Autodesk Inventor part; units mm, degrees
ref_plane "YZ Plane" through (0, 0, 0) normal (1, 0, 0) x (0, 1, 0)
ref_plane "XZ Plane" through (0, 0, 0) normal (0, 1, 0) x (-1, 0, 0)
ref_plane "XY Plane" through (0, 0, 0) normal (0, 0, 1) x (1, 0, 0)
sketch "face_sketch" plane through (0, 0, 0) normal (0, 1, 0) x (-1, 0, 0)
  line L0 (0, 0) -> (25.4, 0)
  line L1 (25.4, 0) -> (25.4, -127)
  line L2 (25.4, -127) -> (0, -127)
  line L3 (0, -127) -> (0, 0)
  line L4 (25.4, -50.8) -> (152.4, -50.8)
  line L5 (152.4, -50.8) -> (152.4, -76.2)
  line L6 (152.4, -76.2) -> (25.4, -76.2)
  line L7 (25.4, -76.2) -> (25.4, -50.8)
  line L8 (152.4, -50.8) -> (25.4, 0)
  line L9 (152.4, -76.2) -> (25.4, -127)
  dimension "d0" = 25.4
  dimension "d1" = 127
  dimension "d2" = 127
  dimension "d3" = 25.4
extrude "Plate1" add sketch "face_sketch" along normal blind 3.048
sketch "rivet_holes_sketch" plane through (0, 3.048, 0) normal (0, 1, 0) x (1, 0, 0)
  line L0 (-25.4, 0) -> (-152.4, 50.8)
  line L1 (0, 0) -> (-25.4, 0)
  line L2 (0, 127) -> (0, 0)
  line L3 (-25.4, 127) -> (0, 127)
  line L4 (-152.4, 76.2) -> (-25.4, 127)
  line L5 (-152.4, 50.8) -> (-152.4, 76.2)
  line L6 (-25.4, 127) -> (-25.4, 0) construction
  line L7 (0, 127) -> (-25.4, 127) construction
  line L8 (-25.4, 0) -> (0, 0) construction
  line L9 (-152.4, 76.2) -> (-152.4, 50.8) construction
  line L10 (-152.4, 63.5) -> (-131.2333, 63.5) construction
  line L11 (-131.2333, 63.5) -> (-110.0667, 63.5) construction
  line L12 (-110.0667, 63.5) -> (-88.9, 63.5) construction
  line L13 (-88.9, 63.5) -> (-67.7333, 63.5) construction
  line L14 (-67.7333, 63.5) -> (-46.5667, 63.5) construction
  line L15 (-46.5667, 63.5) -> (-25.4, 63.5) construction
  line L16 (-12.7, 0) -> (-12.7, 21.1667) construction
  line L17 (-12.7, 21.1667) -> (-12.7, 42.3333) construction
  line L18 (-12.7, 42.3333) -> (-12.7, 63.5) construction
  line L19 (-12.7, 63.5) -> (-12.7, 84.6667) construction
  line L20 (-12.7, 84.6667) -> (-12.7, 105.8333) construction
  line L21 (-12.7, 105.8333) -> (-12.7, 127) construction
hole "rivet_holes" at (-131.2333, 3.048, -63.5) at (-110.0667, 3.048, -63.5) at (-88.9, 3.048, -63.5) at (-67.7333, 3.048, -63.5) at (-46.5667, 3.048, -63.5) at (-12.7, 3.048, -21.1667) at (-12.7, 3.048, -42.3333) at (-12.7, 3.048, -63.5) at (-12.7, 3.048, -84.6667) at (-12.7, 3.048, -105.8333) direction (0, -1, 0) diameter 3.5719 depth 3.048 tip angle 118
sketch "hm_mounting_slot_sketch" plane through (0, 3.048, 0) normal (0, 1, 0) x (1, 0, 0)
  line L0 (-67.437, 87.503) -> (-26.797, 87.503) construction
  line L1 (-67.437, 88.9) -> (-26.797, 88.9)
  line L2 (-26.797, 86.106) -> (-67.437, 86.106)
  arc A0 (-67.437, 88.9) -> (-67.437, 86.106) centre (-67.437, 87.503) ccw
  arc A1 (-26.797, 86.106) -> (-26.797, 88.9) centre (-26.797, 87.503) ccw
  line L3 (-67.437, 39.497) -> (-26.797, 39.497) construction
  line L4 (-67.437, 38.1) -> (-26.797, 38.1)
  line L5 (-26.797, 40.894) -> (-67.437, 40.894)
  arc A2 (-67.437, 40.894) -> (-67.437, 38.1) centre (-67.437, 39.497) ccw
  arc A3 (-26.797, 38.1) -> (-26.797, 40.894) centre (-26.797, 39.497) ccw
  line L6 (-25.4, 0) -> (-25.4, 127) construction
  line L7 (-68.834, 87.503) -> (-68.834, 109.6264) construction
  line L8 (-25.4, 127) -> (-152.4, 76.2)
  line L9 (-68.834, 39.497) -> (-68.834, 17.3736) construction
  line L10 (-152.4, 50.8) -> (-25.4, 0)
  point P0 (0, 0)
  point P1 (-47.117, 87.503)
  point P2 (-47.117, 39.497)
  point P3 (-25.4, 39.497)
  point P4 (-25.4, 87.503)
  point P5 (-68.834, 28.4353)
  dimension "d12" = 40.64
  dimension "d14" = 2.794
  dimension "d15" = 40.64
  dimension "d16" = 2.794
  dimension "d17" = 50.8
extrude "Cut1" cut sketch "hm_mounting_slot_sketch" against normal blind 3.048
equation "\"d5\" = rv_hole_diameter"
equation "\"d10\" = Thickness"
equation "\"d12\" = tb_hm_mounting_slot_length"
equation "\"d15\" = tb_hm_mounting_slot_length"
equation "\"d17\" = hm_base_length"
equation "\"d18\" = Thickness"
equation "\"d0\" = st_outer_diameter"
equation "\"d1\" = tb_rivet_row_length"
equation "\"d2\" = tb_rivet_row_length"
equation "\"d3\" = st_outer_diameter"
equation "\"Thickness\" = tb_metal_thickness"
equation "\"BendRadius\" = Thickness"
equation "\"BendReliefWidth\" = Thickness"
equation "\"BendReliefDepth\" = 0.5 * Thickness"
equation "\"CornerReliefSize\" = 4 * Thickness"
equation "\"MinimumRemnant\" = 2 * Thickness"
equation "\"TransitionRadius\" = BendRadius"
equation "\"JacobiRadiusSize\" = BendRadius"
equation "\"GapSize\" = Thickness"
equation "\"bp_thickness\" = 3.048"
equation "\"bp_height\" = gb_mh_seperation + st_outer_diameter"
equation "\"bp_width\" = 4 * st_rivet_distance"
equation "\"bp_axle_height\" = magic_axle_offset + gb_axle_from_edge + gb_to_bottom_of_side_assembly"
equation "\"magic_axle_offset\" = 2.286"
equation "\"bp_tensioner_width\" = 6.35"
equation "\"bp_tensioner_height\" = 50.8"
equation "\"bp_tensioner_from_bottom\" = 38.1"
equation "\"bp_tensioner_from_side\" = 25.4"
equation "\"bp_tensioner_wood_mount_from_tensioner_top\" = 12.7"
equation "\"bp_tensioner_wood_mount_diameter\" = 6.35"
equation "\"gb_mh_seperation\" = 111.1504"
equation "\"gb_mh_diameter\" = 6.35"
equation "\"gb_axle_from_edge\" = 38.1"
equation "\"gb_width\" = 127"
equation "\"gb_bearing_diameter\" = 28.575"
equation "\"gb_to_bottom_of_side_assembly\" = 4.7752"
equation "\"rv_hole_diameter\" = 3.57187"
equation "\"st_outer_diameter\" = 25.4"
equation "\"st_wall_thickness\" = 1.5875"
equation "\"st_length\" = 685.8"
equation "\"st_gbmh_from_center\" = 0.5 * gb_mh_seperation"
equation "\"st_cutout_depth_right\" = 203.2"
equation "\"st_cutout_depth_left\" = 203.2"
equation "\"st_rivet_distance\" = 19.05"
equation "\"so_inner_diameter\" = 7.62"
equation "\"so_wall_thickness\" = 5.08"
equation "\"so_length\" = 40.64"
equation "\"twb_width\" = st_outer_diameter"
equation "\"twb_length\" = bp_tensioner_width + 2 * twb_margin_on_each_side"
equation "\"twb_height\" = 2 * bp_tensioner_wood_mount_diameter + bp_tensioner_height + 2 * bp_tensioner_wood_mount_from_tensioner_top + twb_margin_on_each_side"
equation "\"twb_margin_on_each_side\" = 6.35"
equation "\"twb_tensioner_from_edge\" = -0.5 * bp_tensioner_height + 0.5 * twb_height"
equation "\"tb_side_length\" = 127"
equation "\"tb_rivet_row_length\" = 127"
equation "\"d4\" = BendRadius"
equation "\"tb_metal_thickness\" = 3.048"
equation "\"tb_hm_mounting_slot_length\" = 40.64"
equation "\"hm_base_width\" = 30.48"
equation "\"hm_base_length\" = 50.8"
equation "\"hm_moon_flange_radius\" = 17.78"
equation "\"hm_moon_channel_offset\" = 2.286"
equation "\"hm_moon_flange_width\" = 5.08"
equation "\"hm_moon_thickness\" = 5.08"
equation "\"hm_base_height\" = 5.08"
equation "\"hm_peg_width\" = 2.54"
equation "\"hm_peg_length\" = 5.08"
equation "\"hm_peg_height\" = 5.08"
equation "\"hm_rivet_groove_width\" = 10.16"
equation "\"hm_rivet_groove_height\" = 1.27"
equation "\"gb_mh_seperation_alt\" = 111.125"
equation "\"gb_axle_from_edge_alt\" = 43.1546"
equation "\"bp_axle_height_alt\" = magic_axle_offset + gb_axle_from_edge_alt + gb_to_bottom_of_side_assembly"
properties part number "traingle_bracket(tb)" material "Aluminum 6061"
Source: CAD feature listing. Evaluate the final solid. Frame: model axes, mm. A direction names the side the tool comes from. Round coordinates to 2 decimals unless told otherwise and drop trailing zeros. Order: outer loops, then holes, each group sorted by start corner. A loop starts at its lowest first (then second) coordinate and runs counter-clockwise, first axis right, second up. Notation, with made-up numbers: (-26, 46.25) -> (17, 46.25) arc R33 cw to (17, 75.25) -> close; hole circle Ø4 at (-38, -2). An arc over 180 degrees is marked (long way). Answer as CSV lines item,"result".
Item 1: Pull-direction query (X, two-part tool) for faces 3 (the face through (-89.789, 1.503, -101.244)), 4 (the face through (-13.236, 1.503, -82.963)), 5 (the face through (-14.206, 1.503, -104.873)), 6 (the face through (-58, 0, -63)); classes: pulls with the +X half, pulls with the -X half, needs draft (parallel to the pull), parting line crosses it, or undercut.
A:
face 3,"pulls with the -X half"
face 4,"undercut"
face 5,"undercut"
face 6,"needs draft"
Item 2: Section D-D, the plane x = -41.5. Return loops of the section in (y, z), plus the area to 3 significant figures.
A:
outline,"(0, -120.56) -> (3.05, -120.56) -> (3.05, -88.9) -> (0, -88.9) -> close; (0, -86.11) -> (3.05, -86.11) -> (3.05, -40.89) -> (0, -40.89) -> close; (0, -38.1) -> (3.05, -38.1) -> (3.05, -6.44) -> (0, -6.44) -> close"
area,"331 mm²"
Item 3: Section A-A, the plane z = -63.5. Return loops of the section in (x, y), plus the area to 3 significant figures.
A:
outline,"(-152.4, 0) -> (-133.02, 0) -> (-133.02, 3.05) -> (-152.4, 3.05) -> close; (-129.45, 0) -> (-111.85, 0) -> (-111.85, 3.05) -> (-129.45, 3.05) -> close; (-108.28, 0) -> (-90.69, 0) -> (-90.69, 3.05) -> (-108.28, 3.05) -> close; (-87.11, 0) -> (-69.52, 0) -> (-69.52, 3.05) -> (-87.11, 3.05) -> close; (-65.95, 0) -> (-48.35, 0) -> (-48.35, 3.05) -> (-65.95, 3.05) -> close; (-44.78, 0) -> (-14.49, 0) -> (-14.49, 3.05) -> (-44.78, 3.05) -> close; (-10.91, 0) -> (0, 0) -> (0, 3.05) -> (-10.91, 3.05) -> close"
area,"399 mm²"
Item 4: Line query: L1, parallel to Z at x = -12.7, y = 2.2; L2, parallel to Z at x = -65, y = 1.7; L3, parallel to Z at x = -67, y = 2.8. Output: solid intervals per line, ascending.
A:
L1,"-127 to -107.62, -104.05 to -86.45, -82.88 to -65.29, -61.71 to -44.12, -40.55 to -22.95, -19.38 to 0"
L2,"-111.16 to -88.9, -86.11 to -40.89, -38.1 to -15.84"
L3,"-110.36 to -88.9, -86.11 to -65.13, -61.87 to -40.89, -38.1 to -16.64"
Item 5: Pin query (flat end, axial travel): pin 1 Ø3 at (x, z) = (-46.57, -63.5) entering from +Y; pin 2 Ø0.9 at (x, y) = (-42.5, 1) entering from +Z; pin 3 Ø0.9 at (x, y) = (-47.5, 2) entering from -Z. Return the tip coordinate at first contact, or that it passes through.
A:
pin 1,"through"
pin 2,"z = -6.66"
pin 3,"z = -118.34"
Item 6: Section B-B, the plane x = -88.9. Return loops of the section in (y, z), plus the area to 3 significant figures.
A:
outline,"(0, -101.6) -> (3.05, -101.6) -> (3.05, -65.29) -> (0, -65.29) -> close; (0, -61.71) -> (3.05, -61.71) -> (3.05, -25.4) -> (0, -25.4) -> close"
area,"221 mm²"
Item 7: Section C-C, the plane x = -12.7. Return loops of the section in (y, z), plus the area to 3 significant figures.
A:
outline,"(0, -127) -> (3.05, -127) -> (3.05, -107.62) -> (0, -107.62) -> close; (0, -104.05) -> (3.05, -104.05) -> (3.05, -86.45) -> (0, -86.45) -> close; (0, -82.88) -> (3.05, -82.88) -> (3.05, -65.29) -> (0, -65.29) -> close; (0, -61.71) -> (3.05, -61.71) -> (3.05, -44.12) -> (0, -44.12) -> close; (0, -40.55) -> (3.05, -40.55) -> (3.05, -22.95) -> (0, -22.95) -> close; (0, -19.38) -> (3.05, -19.38) -> (3.05, 0) -> (0, 0) -> close"
area,"333 mm²"
Item 8: Reachability of faces 1 (the face through (-47, 2, -86.106)), 2 (the face through (-58, 3.048, -63)) from +Z, -Z, +X, -X, +Y, -Y: full face, straight path, thin tool, end or side. Return the list, or none.
A:
face 1,"+Y, -Y"
face 2,"+Z, -Z, +X, -X, +Y"
